Verification items for the finished model (mm, model axes). A direction names the side the tool comes from. Give positions to 0.01 mm unless a question says otherwise; leave off trailing zeros. Loops run counter-clockwise (first coordinate to the right, second up) from the corner with the lowest first, then second, coordinate; pieces in that order, holes last. Notation, with made-up numbers: M 35,-13.5 L 79,-13.5 A29 ccw 79,17.5 Z; hole C -30.75,35 d4. An arc over 180 degrees is marked long. Use a Markdown table: item, result.
from build123d import *

# Parameters (mm, degrees)
F0_W           = 254
F0_H           = 76.2
F1_DEPTH       = 50.8
F2_D           = 11.5062
F2_DEPTH       = 19.05
F2_TIP         = 3.4568112273
F4_D           = 12.7
F4_DEPTH       = 228.6
F4_CBORE_D     = 19.05
F4_CBORE_DEPTH = 25.4
F4_TIP         = 3.8154649308


with BuildPart() as f1:
    # F0 (on Top) → F1 (new body)
    with BuildSketch(Plane.XY):
        Rectangle(F0_W, F0_H)
    extrude(amount=-F1_DEPTH)

    # F2
    with Locations(Plane.XY):
        with Locations((-50.8, 19.05), (50.8, 19.05), (50.8, -19.05), (-50.8, -19.05)):
            Hole(F2_D / 2, depth=F2_DEPTH)
            with Locations((0, 0, -(F2_DEPTH + F2_TIP / 2))):  # 118° drill point
                Cone(0, F2_D / 2, F2_TIP, mode=Mode.SUBTRACT)

    # F4
    with Locations(Plane.YZ.offset(127)):
        with Locations((0, -25.4)):
            CounterBoreHole(F4_D / 2, F4_CBORE_D / 2, F4_CBORE_DEPTH, depth=F4_DEPTH)
            with Locations((0, 0, -(F4_DEPTH + F4_TIP / 2))):  # 118° drill point
                Cone(0, F4_D / 2, F4_TIP, mode=Mode.SUBTRACT)


solid = f1.part
(1) Set-up check for faces 5 (the cylindrical face through (52.047, 13.434, -9.658)), 6 (the flat face through (101.6, 2, -32)), 7 (the flat face through (-127, -1, -25)): record each of +Z, -Z, +X, -X, +Y, -Y from which the full face is reachable in a straight line by a thin tool's end or side.
Results below:
| item | result |
|---|---|
| face 5 | +Z |
| face 6 | +X |
| face 7 | +Z, -Z, -X, +Y, -Y |
(2) Draft check along X on faces 1 (the conical face through (49.802, -19.006, -21.906)), 2 (the cylindrical face through (-1.42, 1.38, -31.6)), 3 (the conical face through (-104.75, -0.24, -26.48)), 4 (the conical face through (-49.88, 18.67, -21.91)). Enter one of: +X half, -X half, draft (parallel to the pull), parting line (faces both ways), or undercut.
Results below:
| item | result |
|---|---|
| face 1 | undercut |
| face 2 | draft |
| face 3 | +X half |
| face 4 | undercut |
(3) Cross-section at B-B on x = 106.5. Record the cut outline in (y, z) (3 decimals).
Results below:
| item | result |
|---|---|
| outline | M -38.1,-50.8 L 38.1,-50.8 L 38.1,0 L -38.1,0 Z; hole C 0,-25.4 d19.05 |
(4) Material ranges on line 1 (Y direction, x = -50.8, z = -13.5); line 2 (X direction, y = -19.05, z = -14); line 3 (Y direction, x = 56, z = -8), recorded low to high.
Results below:
| item | result |
|---|---|
| line 1 | -38.1 to -24.8, -13.3 to 13.3, 24.8 to 38.1 |
| line 2 | -127 to -56.55, -45.05 to 45.05, 56.55 to 127 |
| line 3 | -38.1 to -21.51, -16.59 to 16.59, 21.51 to 38.1 |
(5) Cross-section at A-A on z = -6. Record the cut outline in (x, y).
Results below:
| item | result |
|---|---|
| outline | M -127,-38.1 L 127,-38.1 L 127,38.1 L -127,38.1 Z; hole C -50.8,-19.05 d11.51; hole C -50.8,19.05 d11.51; hole C 50.8,-19.05 d11.51; hole C 50.8,19.05 d11.51 |
(6) Gauge pin test, flat ends, axial feed: P1, Ø7, axis at x = 50.8, y = -19.05, coming from the +Z side; P2, Ø5.5, axis at y = 1.5, z = -22, coming from the +X side; P3, Ø10.5, axis at x = -50.8, y = 19.05, coming from the +Z side; P4, Ø10, axis at x = 89.5, y = -19, coming from the +Z side. Record the tip position at first contact, or that the pin passes through.
Results below:
| item | result |
|---|---|
| P1 | z = -20.4 |
| P2 | x = 101.6 |
| P3 | z = -19.35 |
| P4 | z = 0 |
(7) Cross-section at C-C on x = 8.5. Record the cut outline in (y, z), then the cut area to 3 significant figures.
Results below:
| item | result |
|---|---|
| outline | M -38.1,-50.8 L 38.1,-50.8 L 38.1,0 L -38.1,0 Z; hole C 0,-25.4 d12.7 |
| area | 3,740 mm^2 |
